```python
from build123d import *

# Parameters (mm, degrees)
F1_DEPTH = 76.2
F2_R     = 12.7
F3_DEPTH = 76.201
F4_W     = 12.7
F4_H     = 25.4
F5_DEPTH = 25.401
F6_R     = 38.1


with BuildPart() as f1:
    # F0 (on Front) → F1 (new body, symmetric)
    with BuildSketch(Plane.XZ):
        Polygon((-76.2, 25.4), (-76.2, 0), (0, 0), (0, 152.4), (-25.4, 152.4), (-25.4, 25.4), align=None)
    extrude(amount=F1_DEPTH, both=True)

    # F2 (on face) → F3 (cut, through all)
    with BuildSketch(Plane.YZ):
        with Locations((0, 114.3)):
            Circle(F2_R)
    extrude(amount=-F3_DEPTH, mode=Mode.SUBTRACT)

    # F4 (on face) → F5 (cut, through all)
    with BuildSketch(Plane.XY.offset(25.4)):
        with Locations((-69.85, 0)):
            Rectangle(F4_W, F4_H)
        with BuildLine():
            ThreePointArc((-63.5, -12.7), (-50.8, 0), (-63.5, 12.7))
            Line((-63.5, 12.7), (-63.5, -12.7))
        make_face()
    extrude(amount=-F5_DEPTH, mode=Mode.SUBTRACT)

    # F6
    f6_edges = [f1.edges().sort_by_distance(p)[0] for p in [
        (-12.7, 76.2, 152.4),
        (-12.7, -76.2, 152.4),
    ]]
    fillet(f6_edges, radius=F6_R)


solid = f1.part
```
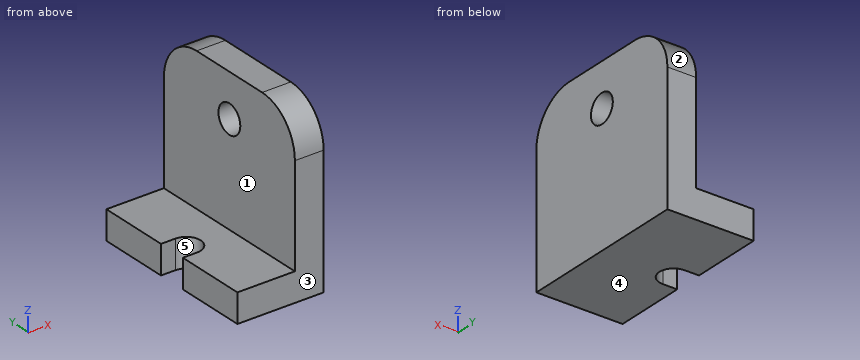
Geometry: final body of the model. Coordinates: model frame, mm. Face numbers are marked on the shaded views. A direction names the side the tool comes from. Coordinates: 2 decimals unless noted, no trailing zeros. Loops run counter-clockwise (first coordinate to the right, second up) from the corner with the lowest first, then second, coordinate; pieces in that order, holes last. Notation, with made-up numbers: (29, 81) -> (64, 81) arc R35 ccw to (64, 113) -> close; hole circle Ø8 at (20.5, 46). An arc over 180 degrees is marked (long way). Use a Markdown table: item, result. Add a question column.
(1) Section query B-B, the plane y = 0. Return loops of the section in (x, z).
(2) Pin query (flat end, axial travel): pin 1 Ø15 at (y, z) = (0, 114.3) entering from -X; pin 2 Ø1.5 at (y, z) = (28, 71) entering from -X; pin 3 Ø4 at (x, y) = (-45.5, 5.5) entering from +Z. Return the tip coordinate at first contact, or that it passes through.
(3) Access query for the marked faces 1 and 2. Directions: +Z, -Z, +X, -X, +Y, -Y. A direction counts if a zero-diameter tool reaches every point of the face in a straight line with its end or side. Return the directions, or none.
(4) Section query A-A, the plane x = -21.5. Return loops of the section in (y, z), plus the area to 3 significant figures.
(5) Mould query, pull axis Y, two halves, no side actions, for the marked faces 3, 4 and 5. Classes: pulls with the +Y half, pulls with the -Y half, needs draft (parallel to the pull), parting line crosses it, or undercut.
(6) Line query: line 1 along Z through (x, y) = (-10, 0); line 2 along Y through (x, z) = (-7, 114); line 3 along X through (y, z) = (-24, 126). Output: solid intervals per line, ascending.
(7) Section query C-C, the plane z = 122. Return loops of the section in (x, y).
(8) Section query D-D, the plane x = -60.5. Return loops of the section in (y, z).
Answer:
| question | item | result |
|---|---|---|
| 1 | outline | (-50.8, 0) -> (0, 0) -> (0, 101.6) -> (-25.4, 101.6) -> (-25.4, 25.4) -> (-50.8, 25.4) -> close; (-25.4, 127) -> (0, 127) -> (0, 152.4) -> (-25.4, 152.4) -> close |
| 2 | pin 1 | passes through |
| 2 | pin 2 | stops at x = -25.4 |
| 2 | pin 3 | stops at z = 25.4 |
| 3 | face 1 | +Z, -X, +Y, -Y |
| 3 | face 2 | +Z, +X, -X, +Y |
| 4 | outline | (-76.2, 0) -> (76.2, 0) -> (76.2, 114.3) arc R38.1 ccw to (38.1, 152.4) -> (-38.1, 152.4) arc R38.1 ccw to (-76.2, 114.3) -> close; hole circle Ø25.4 at (0, 114.3) |
| 4 | area | 22,100 mm^2 |
| 5 | face 3 | pulls with the -Y half |
| 5 | face 4 | needs draft |
| 5 | face 5 | undercut |
| 6 | line 1 | z = 0 to 101.6, 127 to 152.4 |
| 6 | line 2 | y = -76.2 to -12.7, 12.7 to 76.2 |
| 6 | line 3 | x = -25.4 to 0 |
| 7 | outline | (-25.4, -75.41) -> (0, -75.41) -> (0, -10.1) -> (-25.4, -10.1) -> close; (-25.4, 10.1) -> (0, 10.1) -> (0, 75.41) -> (-25.4, 75.41) -> close |
| 8 | outline | (-76.2, 0) -> (-12.34, 0) -> (-12.34, 25.4) -> (-76.2, 25.4) -> close; (12.34, 0) -> (76.2, 0) -> (76.2, 25.4) -> (12.34, 25.4) -> close |
